CAD build for the part. Positions are in the model's coordinates, mm. Face numbers are marked on the shaded views. A direction names the side the tool comes from. Round coordinates to 2 decimals unless told otherwise and drop trailing zeros.
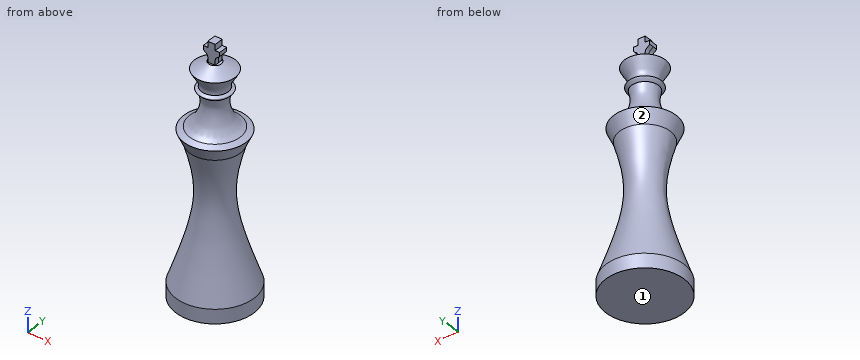
from build123d import *

# Parameters (mm, degrees)
F0_W     = 17.1797536314
F0_H     = 6.2460470638
F2_DEPTH = 2


with BuildPart() as f1:
    # F0 (on Front) → F1 (revolve)
    with BuildSketch(Plane.XZ):
        with Locations((-8.5898768157, -39.7314429283)):
            Rectangle(F0_W, F0_H)
        with BuildLine():
            add(Edge.make_bspline(
                [(-17.1797536314, -36.6084193964), (-13.8412130362, -27.0733219531), (-3.7655602714, -0.1039771833), (-9.60948889, 16.5696096292), (-11.1084822565, 22.6635169238)],
                knots=[0, 0, 0, 0, 0.5622745719, 1, 1, 1, 1], degree=3))
            Line((-17.1797536314, -36.6084193964), (0, -36.6084193964))
            Line((0, -36.6084193964), (0, 57.2025813162))
            Line((0, 57.2025813162), (-1.5886335168, 57.2025813162))
            Line((-1.5886335168, 57.2025813162), (-2.7994840118, 57.2025813162))
            Line((-2.7994840118, 57.2025813162), (-8.9197969064, 54.0465675294))
            add(Edge.make_bspline(
                [(-5.8707841672, 46.6392822564), (-5.2688373253, 49.3856109679), (-7.9407452916, 51.5203798811), (-8.9197969064, 54.0465675294)],
                knots=[0, 0, 0, 0, 8.0102655262, 8.0102655262, 8.0102655262, 8.0102655262], degree=3))
            add(Edge.make_bspline(
                [(-5.8707841672, 44.4355420768), (-6.4785506158, 44.8487001919), (-7.9604304678, 46.1172039826), (-6.4081557233, 46.3077279426), (-5.8707841672, 46.6392822564)],
                knots=[0, 0, 0, 0, 0.5323422757, 1, 1, 1, 1], degree=3))
            add(Edge.make_bspline(
                [(-11.1084822565, 29.491815716), (-7.8871886606, 31.232032236), (-4.125628446, 39.4230942254), (-5.5170923569, 42.2844330979), (-5.8707841672, 44.4355420768)],
                knots=[0, 0, 0, 0, 0.5894302475, 1, 1, 1, 1], degree=3))
            Line((-11.1084822565, 29.491815716), (-13.6886807159, 28.3834971488))
            Line((-13.6886807159, 28.3834971488), (-11.1084822565, 22.6635169238))
        make_face()
    revolve(axis=Axis((0, 0, 4.9645396212), (0, 0, -1)))

    # F0 (on Front) → F2 (join, symmetric)
    with BuildSketch(Plane.XZ):
        with BuildLine():
            Line((-1.5886335168, 57.2025813162), (0, 57.2025813162))
            Line((0, 57.2025813162), (0, 66.1251172423))
            Line((0, 66.1251172423), (-1.62465428, 66.1251172423))
            Line((-1.62465428, 66.1251172423), (-1.62465428, 63.5033920407))
            Line((-1.62465428, 63.5033920407), (-3.6026129965, 63.5033920407))
            Line((-3.6026129965, 63.5033920407), (-3.6026129965, 61.8110969663))
            add(Edge.make_bspline(
                [(-1.5886335168, 57.2025813162), (-1.498904641, 58.1154281999), (-1.381835571, 60.6809226763), (-3.1117708882, 61.128619796), (-3.6026129965, 61.8110969663)],
                knots=[0, 0, 0, 0, 0.5359349994, 1, 1, 1, 1], degree=3))
        make_face()
        with BuildLine():
            Line((0, 66.1251172423), (0, 57.2025813162))
            Line((0, 57.2025813162), (1.5886335168, 57.2025813162))
            add(Edge.make_bspline(
                [(1.5886335168, 57.2025813162), (1.498904641, 58.1154281999), (1.381835571, 60.6809226763), (3.1117708882, 61.128619796), (3.6026129965, 61.8110969663)],
                knots=[0, 0, 0, 0, 0.5359349994, 1, 1, 1, 1], degree=3))
            Line((3.6026129965, 61.8110969663), (3.6026129965, 63.5033920407))
            Line((3.6026129965, 63.5033920407), (1.62465428, 63.5033920407))
            Line((1.62465428, 63.5033920407), (1.62465428, 66.1251172423))
            Line((1.62465428, 66.1251172423), (0, 66.1251172423))
        make_face()
    extrude(amount=F2_DEPTH, both=True)


solid = f1.part
Item 1: 3-axis set-ups, long thin cutter, end or side, ignore diameter. For the marked faces 1 and 2: which of +Z, -Z, +X, -X, +Y, -Y reach the whole face in a straight line?
Verdict:
face 1: -Z, +X, -X, +Y, -Y
face 2: none
Item 2: Flat gauge pins, fed straight in: P1, Ø12, axis at y = 10, z = -27.5, coming from the +X side; P2, Ø1.5, axis at x = 4.5, y = -5.5, coming from the +Z side; P3, Ø2, axis at y = 0.5, z = 65, coming from the -X side; P4, Ø5, axis at y = -10.5, z = 3.5, coming from the -X side. Where does each tip first touch, or does it go through?
Verdict:
P1: stops at x = 14.36
P2: stops at z = 55.37
P3: stops at x = -1.62
P4: passes through
Item 3: Cut at A-A (x = 6). State how many separate pieces and enclosed holes the cut face has, plus the area to 3 significant figures.
Verdict:
separate pieces: 3
enclosed holes: 0
area: 1,470 mm2
